Geometry check sheet. Reference: the model listing, model coordinates, mm. A direction names the side the tool comes from. Coordinates: 2 decimals unless noted, no trailing zeros. Write each loop counter-clockwise with the first axis right and the second up, starting at its lowest first coordinate (ties: lowest second). Pieces come first, ordered by that corner, then holes. Notation, with made-up numbers: (18, 31.5) - (34, 31.5) arc R24 cw to (34, 65.5) - close; hole circle Ø10 at (70.5, -3). An arc over 180 degrees is marked (long way). Answer as a JSON object with one key per item and string values. Group by question number.
from build123d import *

# Parameters (mm, degrees)
SKETCH7_W           = 40
SKETCH7_H           = 40
BOSS_EXTRUDE1_DEPTH = 14
LOFT1_START         = -20
LOFT1_DEPTH         = 40
SKETCH16_W          = 49.026286786
SKETCH16_H          = 65.242270374
SKETCH16_R          = 20
CUT_EXTRUDE3_DEPTH  = 6
SKETCH17_W          = 40
SKETCH17_H          = 8
BOSS_EXTRUDE5_DEPTH = 18
SKETCH10_R          = 2.25
CUT_EXTRUDE1_DEPTH  = 25
CHAMFER1_SIZE       = 2.5
FILLET3_R           = 20
SKETCH11_W          = 60
SKETCH11_H          = 18
BOSS_EXTRUDE6_DEPTH = 90
FILLET9_R           = 2.5
SKETCH20_W          = 50
SKETCH20_H          = 8
CUT_EXTRUDE4_DEPTH  = 80
SKETCH28_W          = 15
SKETCH28_H          = 8
BOSS_EXTRUDE7_DEPTH = 10
FILLET13_R          = 4
SKETCH37_W          = 60
SKETCH37_H          = 90
CUT_EXTRUDE8_DEPTH  = 5
FILLET16_R          = 5
SKETCH38_R          = 1.7
CUT_EXTRUDE9_DEPTH  = 22
CHAMFER3_SIZE       = 1.6


# Read off the part's stored shape, not the designer's step: Loft1
with BuildPart() as part:
    # Sketch7 → Boss-Extrude1 (new body)
    with BuildSketch(Plane.XY):
        Rectangle(SKETCH7_W, SKETCH7_H)
    extrude(amount=BOSS_EXTRUDE1_DEPTH)

    # Loft1 outline → Loft1 (add)
    with BuildSketch(Plane.YZ.offset(LOFT1_START)):
        with BuildLine():
            add(Edge.make_bspline(
                [(-38, 18), (-31.853637028, 18), (-26.146362972, 14), (-20, 14)],
                knots=[0, 0, 0, 0, 1, 1, 1, 1], degree=3))
            Line((-38, 18), (-38, 10))
            add(Edge.make_bspline(
                [(-38, 10), (-31.853637028, 10), (-26.146362972, 6), (-20, 6)],
                knots=[0, 0, 0, 0, 1, 1, 1, 1], degree=3))
            Line((-20, 6), (-20, 14))
        make_face()
    extrude(amount=LOFT1_DEPTH)

    # Sketch16 → Cut-Extrude3 (cut)
    with BuildSketch(Plane(origin=(0, 0, 0), x_dir=(-1, 0, 0), z_dir=(0, 0, -1))):
        Rectangle(SKETCH16_W, SKETCH16_H)
        Circle(SKETCH16_R, mode=Mode.SUBTRACT)
    extrude(amount=-CUT_EXTRUDE3_DEPTH, mode=Mode.SUBTRACT)

    # Sketch17 → Boss-Extrude5 (add)
    with BuildSketch(Plane(origin=(0, -38, 0), x_dir=(-1, 0, 0), z_dir=(0, -1, 0))):
        with Locations((0, -14)):
            Rectangle(SKETCH17_W, SKETCH17_H)
    extrude(amount=BOSS_EXTRUDE5_DEPTH)

    # Sketch10 → Cut-Extrude1 (cut)
    with BuildSketch(Plane.XY.offset(14)):
        with Locations((-7.00009521, 12.124420806)):
            Circle(SKETCH10_R)
        with Locations((6.99990479, 12.124420806)):
            Circle(SKETCH10_R)
        with Locations((13.99990479, 6.5153e-05)):
            Circle(SKETCH10_R)
        with Locations((6.99990479, -12.1242905)):
            Circle(SKETCH10_R)
        with Locations((-7.00009521, -12.1242905)):
            Circle(SKETCH10_R)
        with Locations((-14.00009521, 6.5153e-05)):
            Circle(SKETCH10_R)
    extrude(amount=-CUT_EXTRUDE1_DEPTH, mode=Mode.SUBTRACT)

    # Chamfer1
    chamfer1_edges = [part.edges().sort_by_distance(p)[0] for p in [
        (4.74990479, 12.124420806, 14),
        (-9.25009521, 12.124420806, 14),
        (-16.25009521, 6.5153e-05, 14),
        (-9.25009521, -12.1242905, 14),
        (4.74990479, -12.1242905, 14),
        (11.74990479, 6.5153e-05, 14),
    ]]
    chamfer(chamfer1_edges, length=CHAMFER1_SIZE)

    # Fillet3
    fillet3_edges = [part.edges().sort_by_distance(p)[0] for p in [
        (20, 20, 10),
        (-20, 20, 10),
    ]]
    fillet(fillet3_edges, radius=FILLET3_R - 0.0001)  # a hair under: the kernel refuses the full size

    # Sketch11 → Boss-Extrude6 (add)
    with BuildSketch(Plane(origin=(0, -56, -3.472963553), x_dir=(1, 0, 0), z_dir=(0, 1, 0))):
        with Locations((0, -12.472963553)):
            Rectangle(SKETCH11_W, SKETCH11_H)
    extrude(amount=-BOSS_EXTRUDE6_DEPTH)

    # Fillet9
    fillet9_edges = [part.edges().sort_by_distance(p)[0] for p in [
        (0, -56, 10),
        (-20, -56, 14),
        (20, -56, 14),
    ]]
    fillet(fillet9_edges, radius=FILLET9_R)

    # Sketch20 → Cut-Extrude4 (cut)
    with BuildSketch(Plane.XZ.offset(146)):
        with Locations((0, 9)):
            Rectangle(SKETCH20_W, SKETCH20_H)
    extrude(amount=-CUT_EXTRUDE4_DEPTH, mode=Mode.SUBTRACT)

    # Sketch28 → Boss-Extrude7 (add)
    with BuildSketch(Plane(origin=(0, -146, 0), x_dir=(-1, 0, 0), z_dir=(0, -1, 0))):
        with Locations((17.5, -9)):
            Rectangle(SKETCH28_W, SKETCH28_H)
        with Locations((-17.5, -9)):
            Rectangle(SKETCH28_W, SKETCH28_H)
    extrude(amount=-BOSS_EXTRUDE7_DEPTH)

    # Fillet13
    fillet13_edges = [part.edges().sort_by_distance(p)[0] for p in [
        (-25, -66, 9),
        (25, -66, 9),
        (-25, -136, 9),
        (-10, -136, 9),
        (10, -136, 9),
        (25, -136, 9),
    ]]
    fillet(fillet13_edges, radius=FILLET13_R)

    # Sketch37 → Cut-Extrude8 (cut)
    with BuildSketch(Plane.XY):
        with Locations((0, -101)):
            Rectangle(SKETCH37_W, SKETCH37_H)
    extrude(amount=CUT_EXTRUDE8_DEPTH, mode=Mode.SUBTRACT)

    # Fillet16
    fillet16_edges = [part.edges().sort_by_distance(p)[0] for p in [
        (30, -56, 11.5),
        (30, -146, 11.5),
        (-30, -146, 11.5),
        (-30, -56, 11.5),
    ]]
    fillet(fillet16_edges, radius=FILLET16_R)

    # Sketch38 → Cut-Extrude9 (cut)
    with BuildSketch(Plane.XY):
        with Locations(Location((25, -61, 0), (0, 0, 180))):
            Circle(SKETCH38_R)
        with Locations(Location((-25, -61, 0), (0, 0, 180))):
            Circle(SKETCH38_R)
        with Locations(Location((-25, -141, 0), (0, 0, 180))):
            Circle(SKETCH38_R)
        with Locations(Location((25, -141, 0), (0, 0, 180))):
            Circle(SKETCH38_R)
    extrude(amount=CUT_EXTRUDE9_DEPTH, mode=Mode.SUBTRACT)

    # Chamfer3
    chamfer3_edges = [part.edges().sort_by_distance(p)[0] for p in [
        (26.7, -141, 18),
        (-23.3, -141, 18),
        (-23.3, -61, 18),
        (26.7, -61, 18),
    ]]
    chamfer(chamfer3_edges, length=CHAMFER3_SIZE)


solid = part.part
(1) Draft check along X on faces 6 (the face through (-14.297, 13.986, 10.056)), 7 (the face through (13.986, 14.297, 10.056)), 8 (the face through (0, 0, 0)), 9 (the face through (10, -143, 9)). Enter one of: +X half, -X half, draft (parallel to the pull), parting line (faces both ways), or undercut.
(2) Gauge pin test, flat ends, axial feed: pin 1 (6 mm diameter, centred on x = 7, y = -12.12, fed in from -Z); pin 2 (5.5 mm diameter, centred on x = 18.5, z = 9.5, fed in from +Y); pin 3 (3.5 mm diameter, centred on y = -38, z = 9.5, fed in from +X); pin 4 (10 mm diameter, centred on x = -12, y = -29, fed in from -Z). Record the tip position at first contact, or that the pin passes through.
(3) Material ranges on L1, parallel to X at y = -12, z = 8.75; L2, parallel to X at y = -141, z = 8; L3, parallel to X at y = -60, z = 17, recorded low to high. Write a range as [from, to].
(4) Set-up check for faces 1 (the face through (23.859, -67.203, 9.056)), 2 (the face through (0, -4, 14)), 3 (the face through (16, -15, 6)), 4 (the face through (-4.74, -11.41, 11.62)), 5 (the face through (-24.63, -139.34, 10.62)): record each of +Z, -Z, +X, -X, +Y, -Y from which the full face is reachable in a straight line by a thin tool's end or side.
(5) Section check A-A (y = -114). Record the cut outline in (x, z), and give its area (3 significant figures).
Conclusion:
{
 "1": {"face 6": "-X half", "face 7": "+X half", "face 8": "draft", "face 9": "undercut"},
 "2": {"pin 1": "stops at z = 0", "pin 2": "stops at y = 12.33", "pin 3": "stops at x = 20", "pin 4": "stops at z = 6.5"},
 "3": {"L1": "x = [-20, -9.25], [-4.75, 4.75], [9.25, 20]", "L2": "x = [-30, -26.7], [-23.3, -10], [10, 23.3], [26.7, 30]", "L3": "x = [-29.9, -27.07], [-22.93, 22.93], [27.07, 29.9]"},
 "4": {"face 1": "-Z", "face 2": "+Z, +X, -X, +Y", "face 3": "-Z, +X", "face 4": "+Z", "face 5": "+Z, -Z"},
 "5": {"outline": "(-30, 5) - (-25, 5) - (-25, 13) - (25, 13) - (25, 5) - (30, 5) - (30, 18) - (-30, 18) - close", "area": "380 mm^2"}
}
